```python
from build123d import *

# Parameters (mm, degrees)
SKETCH2_R           = 1.5
BOSS_EXTRUDE1_DEPTH = 4
BOSS_EXTRUDE2_DEPTH = 15
CHAMFER1_SIZE       = 1.6


with BuildPart() as part:
    # Sketch2 → Boss-Extrude1 (new body)
    with BuildSketch(Plane.XY):
        with BuildLine():
            Line((-15, 15), (15, 15))
            ThreePointArc((15, 15), (30, 0), (15, -15))
            Line((15, -15), (-15, -15))
            ThreePointArc((-15, -15), (-30, 0), (-15, 15))
        make_face()
        with Locations((-15, 8)):
            Circle(SKETCH2_R, mode=Mode.SUBTRACT)
        with Locations((-23, 0)):
            Circle(SKETCH2_R, mode=Mode.SUBTRACT)
        with Locations((-15, -8)):
            Circle(SKETCH2_R, mode=Mode.SUBTRACT)
        with Locations((15, -8)):
            Circle(SKETCH2_R, mode=Mode.SUBTRACT)
        with Locations((23, 0)):
            Circle(SKETCH2_R, mode=Mode.SUBTRACT)
        with Locations((15, 8)):
            Circle(SKETCH2_R, mode=Mode.SUBTRACT)
        with BuildLine():
            Line((-15, 4.15), (15, 4.15))
            ThreePointArc((15, 4.15), (19.15, 0), (15, -4.15))
            Line((15, -4.15), (-15, -4.15))
            ThreePointArc((-15, -4.15), (-19.15, 0), (-15, 4.15))
        make_face(mode=Mode.SUBTRACT)
    extrude(amount=BOSS_EXTRUDE1_DEPTH)

    # Sketch3 → Boss-Extrude2 (add)
    with BuildSketch(Plane.XY.offset(4)):
        with BuildLine():
            Line((-15, -15), (15, -15))
            ThreePointArc((15, -15), (30, 0), (15, 15))
            Line((15, 15), (-15, 15))
            ThreePointArc((-15, 15), (-30, 0), (-15, -15))
        make_face()
        with BuildLine():
            Line((-15, 11.25), (15, 11.25))
            ThreePointArc((15, 11.25), (26.25, 0), (15, -11.25))
            Line((15, -11.25), (-15, -11.25))
            ThreePointArc((-15, -11.25), (-26.25, 0), (-15, 11.25))
        make_face(mode=Mode.SUBTRACT)
    extrude(amount=BOSS_EXTRUDE2_DEPTH)

    # Chamfer1
    chamfer1_edges = [part.edges().sort_by_distance(p)[0] for p in [
        (-16.5, 8, 4),
        (-24.5, 0, 4),
        (-16.5, -8, 4),
        (13.5, -8, 4),
        (21.5, 0, 4),
        (13.5, 8, 4),
    ]]
    chamfer(chamfer1_edges, length=CHAMFER1_SIZE)


solid = part.part
```
The model under review builds one solid part; all positions refer to its coordinate system, in mm. A direction names the side the tool comes from. Round coordinates to 2 decimals unless told otherwise and drop trailing zeros. Write each loop counter-clockwise with the first axis right and the second up, starting at its lowest first coordinate (ties: lowest second). Pieces come first, ordered by that corner, then holes.
(1) We need section B-B on y = 8. Give the boundary of the cut face in (x, z).
(2) Mouldability with a two-part tool opening along Y and no side actions: class faces 1 (the flat face through (0, -15, 9)), 2 (the flat face through (0, 15, 9)), 3 (the flat face through (0, 5, 4)) as +Y half, -Y half, draft (parallel to the pull), parting line (faces both ways), or undercut.
(3) We need section D-D on x = -23. Give the boundary of the cut face in (y, z).
(4) Insertion check: pin 1 (7 mm diameter, centred on x = -7.5, y = -2, fed in from +Z); pin 2 (2.5 mm diameter, centred on x = -15, y = 8, fed in from -Z); pin 3 (1 mm diameter, centred on x = 23.5, z = 6.5, fed in from -Y); pin 4 (2 mm diameter, centred on y = -7, z = 14, fed in from -X). Each pin has a flat end and moves straight along its axis. Give the tip position at first contact, or say it passes through.
(5) Machinability: for faces 4 (the flat face through (0, -11.25, 11)), 5 (the flat face through (0, -4.15, 2)), 6 (the cylindrical face through (30, 0, 9)), which of the approach directions +Z, -Z, +X, -X, +Y, -Y give a long, thin tool a straight path to every point of the face, cutting with its end or side? Answer none if there is none.
(6) We need section C-C on z = 8.5. Give the boundary of the cut face in (x, y).
(7) We need section A-A on x = -10. Give the boundary of the cut face in (y, z), and give its area (3 significant figures).
(8) Wall thickness on L1, parallel to Y at x = 15, z = 0.6; L2, parallel to Y at x = 12.5, z = 1: over which ranges is each line inside the solid? List them lowest first.
Findings below:
1. outline: (-27.69, 0) - (-16.5, 0) - (-16.5, 2.4) - (-18.1, 4) - (-22.91, 4) - (-22.91, 19) - (-27.69, 19) - close; (-13.5, 0) - (13.5, 0) - (13.5, 2.4) - (11.9, 4) - (-11.9, 4) - (-13.5, 2.4) - close; (16.5, 0) - (27.69, 0) - (27.69, 19) - (22.91, 19) - (22.91, 4) - (18.1, 4) - (16.5, 2.4) - close
2. face 1: -Y half
2. face 2: +Y half
2. face 3: undercut
3. outline: (-12.69, 0) - (-1.5, 0) - (-1.5, 2.4) - (-3.1, 4) - (-7.91, 4) - (-7.91, 19) - (-12.69, 19) - close; (1.5, 0) - (12.69, 0) - (12.69, 19) - (7.91, 19) - (7.91, 4) - (3.1, 4) - (1.5, 2.4) - close
4. pin 1: stops at z = 4
4. pin 2: passes through
4. pin 3: stops at y = -12.69
4. pin 4: stops at x = -28.75
5. face 4: +Z
5. face 5: +Z, -Z
5. face 6: +Z, -Z, +X
6. outline: (-15, -15) - (15, -15) arc R15 ccw to (15, 15) - (-15, 15) arc R15 ccw to start; hole (-15, -11.25) - (15, -11.25) arc R11.25 ccw to (15, 11.25) - (-15, 11.25) arc R11.25 ccw to start
7. outline: (-15, 0) - (-4.15, 0) - (-4.15, 4) - (-11.25, 4) - (-11.25, 19) - (-15, 19) - close; (4.15, 0) - (15, 0) - (15, 19) - (11.25, 19) - (11.25, 4) - (4.15, 4) - close
7. area: 199 mm2
8. L1: y = -15 to -9.5, -6.5 to -4.15, 4.15 to 6.5, 9.5 to 15
8. L2: y = -15 to -4.15, 4.15 to 15
